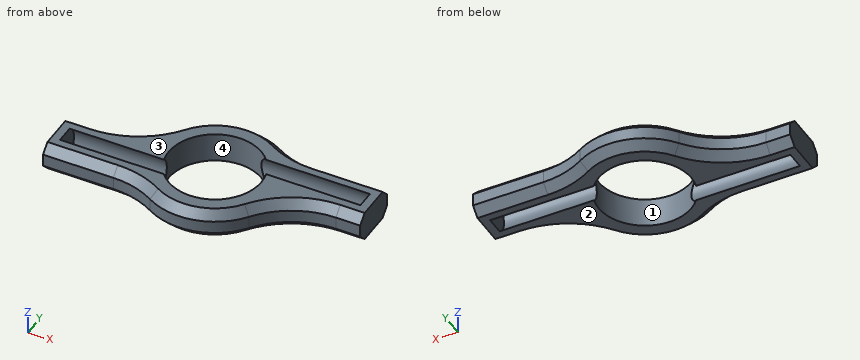
```python
from build123d import *

# Parameters (mm, degrees)
F0_R     = 11
F1_DEPTH = 7
F2_R     = 4.1
F3_DEPTH = 28.8211942778
F4_R     = 4.1
F5_DEPTH = 28.8211942778
F6_W     = 12
F6_H     = 7
F7_DEPTH = 2
F8_W     = 12
F8_H     = 7
F9_DEPTH = 2
F10_R    = 20
F11_SIZE = 2


# Not quite as in the source:
# - a feature names something its author has since deleted; it is built from what else it names


with BuildPart() as f1:
    # F0 (on Top) → F1 (new body)
    with BuildSketch(Plane.XY):
        with BuildLine():
            Line((35, 11), (11.6189500386, 11))
            ThreePointArc((11.6189500386, 11), (-5.4525336701, 15.0422696617), (-15.9687194227, 1))
            Line((-15.9687194227, 1), (-35, 1))
            Line((-35, 1), (-35, -11))
            Line((-35, -11), (-11.6189500386, -11))
            ThreePointArc((-11.6189500386, -11), (5.4525336701, -15.0422696617), (15.9687194227, -1))
            Line((15.9687194227, -1), (35, -1))
            Line((35, -1), (35, 11))
        make_face()
        Circle(F0_R, mode=Mode.SUBTRACT)
    extrude(amount=F1_DEPTH)

    # F2 (on face) → F3 (cut, through all)
    with BuildSketch(Plane.YZ.offset(35)):
        with Locations((5, 3.5)):
            Circle(F2_R)
    extrude(amount=-F3_DEPTH, mode=Mode.SUBTRACT)

    # F4 (on face) → F5 (cut, through all)
    with BuildSketch(Plane(origin=(-35, 0, 0), x_dir=(0, -1, 0), z_dir=(-1, 0, 0))):
        with Locations((5, 3.5)):
            Circle(F4_R)
    extrude(amount=-F5_DEPTH, mode=Mode.SUBTRACT)

    # F6 (on face) → F7 (join)
    with BuildSketch(Plane.YZ.offset(35)):
        with Locations((5, 3.5)):
            Rectangle(F6_W, F6_H)
    extrude(amount=-F7_DEPTH)

    # F8 (on face) → F9 (join)
    with BuildSketch(Plane(origin=(-35, 0, 0), x_dir=(0, -1, 0), z_dir=(-1, 0, 0))):
        with Locations((5, 3.5)):
            Rectangle(F8_W, F8_H)
    extrude(amount=-F9_DEPTH)

    # F10
    f10_edges = [f1.edges().sort_by_distance(p)[0] for p in [
        (11.61895, 11, 3.5),
        (-15.968719, 1, 3.5),
        (15.968719, -1, 3.5),
        (-11.61895, -11, 3.5),
    ]]
    fillet(f10_edges, radius=F10_R)

    # F11
    f11_edges = [f1.edges().sort_by_distance(p)[0] for p in [
        (-26.651503, -11, 7),
        (32.120192, -1, 7),
        (-3.293287, 15.657403, 7),
        (-32.120192, 1, 7),
        (32.120192, -1, 0),
        (-3.293287, 15.657403, 0),
        (-26.651503, -11, 0),
        (-32.120192, 1, 0),
    ]]
    chamfer(f11_edges, length=F11_SIZE)


solid = f1.part
```
Here's how the part is built. I have some questions about the finished solid (model axes, mm). Face numbers are marked on the shaded views. A direction names the side the tool comes from. Round coordinates to 2 decimals unless told otherwise and drop trailing zeros. Order: outer loops, then holes, each group sorted by start corner. A loop starts at its lowest first (then second) coordinate and runs counter-clockwise, first axis right, second up. Notation, with made-up numbers: M -1,37 L 45,37 A29 ccw 45,63 Z; hole C 80.25,-13.75 d6. An arc over 180 degrees is marked long. One line per question, with ' | ' between items.
1) For pin 1 Ø3.5 at (x, z) = (-32.5, 4) entering from +Y; pin 2 Ø0.9 at (x, z) = (-23, 3.5) entering from -Y; pin 3 Ø2 at (y, z) = (4, 4) entering from -X, each with a flat end and sliding along its axis, tell me the tip position at first contact or that it passes through.
Working result:
pin 1: y = 1 | pin 2: y = -11 | pin 3: x = -20.52
2) I want a section at A-A, the plane z = 0.75. Write out the boundary of the cut face in (x, y).
Working result:
outline: M -35,-9.75 L -18.3,-9.75 A21.25 cw -7.5,-12.7 A14.75 ccw 11.98,-8.6 A21.25 cw 29.24,0.25 L 35,0.25 L 35,9.75 L 18.3,9.75 A21.25 cw 7.5,12.7 A14.75 ccw -11.98,8.6 A21.25 cw -29.24,-0.25 L -35,-0.25 Z; hole M -33,-8.04 L -7.51,-8.04 A11 ccw 10.82,1.96 L 33,1.96 L 33,8.04 L 7.51,8.04 A11 ccw -10.82,-1.96 L -33,-1.96 Z
3) I need wall thicknesses on line 1 along X through (y, z) = (-0.5, 2.5); line 2 along Y through (x, z) = (28.5, 5.25); line 3 along X through (y, z) = (-7.5, 1.5). Which ranges of each line are inside material? Lowest first, please.
Working result:
line 1: -35 to -10.99, 10.99 to 35 | line 2: -0.76 to 1.29, 8.71 to 10.75 | line 3: -35 to -33, 8.05 to 13.81
4) For the marked faces 1 and 2, which set-ups out of +Z, -Z, +X, -X, +Y, -Y let a thin tool reach every point of the face, with its end or its side?
Working result:
face 1: +Z, -Z | face 2: -Z, +X, -X, +Y, -Y
5) If we mould it in two halves opening along Y, with no side actions, what happens to the marked faces 3 and 4? For each: +Y half, -Y half, draft (parallel to the pull), parting line (faces both ways), or undercut.
Working result:
face 3: draft | face 4: undercut
